from build123d import *

# Parameters (mm, degrees)
SKETCH1_W           = 32.3
SKETCH1_H           = 36.7
BOSS_EXTRUDE1_DEPTH = 1.5
SKETCH2_W           = 32.3
SKETCH2_H           = 1.5
BOSS_EXTRUDE2_DEPTH = 16.8
SKETCH3_W           = 22.7
SKETCH3_H           = 11.8
BOSS_EXTRUDE3_DEPTH = 3
SKETCH4_R           = 5.9
BOSS_EXTRUDE4_DEPTH = 4.3
SKETCH7_W           = 22.7
SKETCH7_H           = 11.8
BOSS_EXTRUDE6_DEPTH = 3
SKETCH9_R           = 5.9
BOSS_EXTRUDE7_DEPTH = 4.3
BOSS_EXTRUDE8_START = -1.5
SKETCH7_2_W         = 22.7
SKETCH7_2_H         = 11.8
BOSS_EXTRUDE8_DEPTH = 19
BOSS_EXTRUDE9_START = -20.5
SKETCH3_2_W         = 22.7
SKETCH3_2_H         = 11.8
BOSS_EXTRUDE9_DEPTH = 19


with BuildPart() as part:
    # Sketch1 → Boss-Extrude1 (new body)
    with BuildSketch(Plane.XY):
        Rectangle(SKETCH1_W, SKETCH1_H)
    extrude(amount=BOSS_EXTRUDE1_DEPTH)

    # Sketch2 → Boss-Extrude2 (add)
    with BuildSketch(Plane(origin=(0, 0, 0), x_dir=(-1, 0, 0), z_dir=(0, 0, -1))):
        with Locations((0, -17.6)):
            Rectangle(SKETCH2_W, SKETCH2_H)
    extrude(amount=BOSS_EXTRUDE2_DEPTH)

    # Sketch3 → Boss-Extrude3 (add)
    with BuildSketch(Plane.XZ.offset(18.35)):
        with Locations((-0.2, -8.9)):
            Rectangle(SKETCH3_W, SKETCH3_H)
    extrude(amount=BOSS_EXTRUDE3_DEPTH)

    # Sketch4 → Boss-Extrude4 (add)
    with BuildSketch(Plane.XZ.offset(21.35)):
        with BuildLine():
            ThreePointArc((-0.35, -6.307703721), (0.098043145, -7.56958653), (0.25, -8.9))
            ThreePointArc((0.25, -8.9), (0.098043145, -10.23041347), (-0.35, -11.492296279))
            ThreePointArc((-0.35, -11.492296279), (3.85, -8.9), (-0.35, -6.307703721))
        make_face()
        with Locations((-5.65, -8.9)):
            Circle(SKETCH4_R)
    extrude(amount=BOSS_EXTRUDE4_DEPTH)

    # Sketch7 → Boss-Extrude6 (add)
    with BuildSketch(Plane(origin=(-13.214346586, -22.528065204, 1.5), x_dir=(-1, 0, 0), z_dir=(0, 0, 1))):
        with Locations((-13.414346586, -31.978065204)):
            Rectangle(SKETCH7_W, SKETCH7_H)
    extrude(amount=BOSS_EXTRUDE6_DEPTH)

    # Sketch9 → Boss-Extrude7 (add)
    with BuildSketch(Plane(origin=(-13.214346586, -22.528065204, 4.5), x_dir=(-1, 0, 0), z_dir=(0, 0, 1))):
        with Locations((-7.964346586, -31.978065204)):
            Circle(SKETCH9_R)
        with BuildLine():
            ThreePointArc((-13.264346586, -34.570361484), (-13.864346586, -31.978065204), (-13.264346586, -29.385768925))
            ThreePointArc((-13.264346586, -29.385768925), (-17.464346586, -31.978065204), (-13.264346586, -34.570361484))
        make_face()
    extrude(amount=BOSS_EXTRUDE7_DEPTH)

    # Sketch7<2> → Boss-Extrude8 (add)
    with BuildSketch(Plane(origin=(-13.214346586, -22.528065204, 1.5), x_dir=(-1, 0, 0), z_dir=(0, 0, 1)).offset(BOSS_EXTRUDE8_START)):
        with Locations((-13.414346586, -31.978065204)):
            Rectangle(SKETCH7_2_W, SKETCH7_2_H)
    extrude(amount=-BOSS_EXTRUDE8_DEPTH)

    # Sketch3<2> → Boss-Extrude9 (add)
    with BuildSketch(Plane.XZ.offset(18.35).offset(BOSS_EXTRUDE9_START)):
        with Locations((-0.2, -8.9)):
            Rectangle(SKETCH3_2_W, SKETCH3_2_H)
    extrude(amount=BOSS_EXTRUDE9_DEPTH)


solid = part.part
Verification items for the finished model (mm, model axes). A direction names the side the tool comes from. Coordinates: 2 decimals unless noted, no trailing zeros. Loops run counter-clockwise (first coordinate to the right, second up) from the corner with the lowest first, then second, coordinate; pieces in that order, holes last. Notation, with made-up numbers: (14.25, -33) -> (71.25, -33) arc R20 cw to (71.25, -4) -> close; hole circle Ø6 at (89.5, 70). An arc over 180 degrees is marked (long way). Answer as a JSON object with one key per item and string values. Group by question number.
Item 1: Sectioned sample at B-B on x = 7. Record the boundary of the cut face in (y, z), plus the area to 3 significant figures.
Item 2: Tool access check on faces 4 (the flat face through (0, -18, -16.8)), 5 (the flat face through (11.55, 10, -9)), 6 (the cylindrical face through (-11.146, 9.672, 6.62)), 7 (the flat face through (11.15, -20, -9)), 8 (the flat face through (0, -7, -3)). Record the directions out of +Z, -Z, +X, -X, +Y, -Y that give a thin tool (end or side, any length) a straight path to the whole face; none if there is none.
Item 3: Scan lines: probe 1 along Z at (x, y) = (7.5, -5); probe 2 along Y at (x, z) = (4, -7.5); probe 3 along Y at (x, z) = (10.5, -1.5). Record each from-to range of solid material in increasing order.
Item 4: Sectioned sample at D-D on y = 13. Record the boundary of the cut face in (x, z).
Item 5: Sectioned sample at C-C on z = -13.5. Record the boundary of the cut face in (x, y), plus the area to 3 significant figures.
Item 6: Depth check by flat-ended pin: pin 1 (0.9 mm diameter, centred on y = 7, z = 3.5, fed in from -X); pin 2 (2 mm diameter, centred on y = 9, z = -7, fed in from +X); pin 3 (4 mm diameter, centred on x = 8, z = -8.5, fed in from -Y). Enter the tip coordinate at first touch or a pass-through.
Item 7: Sectioned sample at A-A on y = -3.5. Record the boundary of the cut face in (x, z), plus the area to 3 significant figures.
Item 8: Mould release check, pull along Y, two halves, no side actions. Record for faces 1 (the flat face through (0, -7, -14.8)), 2 (the flat face through (4, -21.35, -9)), 3 (the flat face through (0, 9, -19)): +Y half, -Y half, draft (parallel to the pull), parting line (faces both ways), or undercut.
Evaluation:
{
 "1": {"outline": "(-21.35, -14.8) -> (-18.35, -14.8) -> (-18.35, -16.8) -> (-16.85, -16.8) -> (-16.85, -14.8) -> (2.15, -14.8) -> (2.15, -3) -> (-16.85, -3) -> (-16.85, 0) -> (3.55, 0) -> (3.55, -19) -> (15.35, -19) -> (15.35, 0) -> (18.35, 0) -> (18.35, 1.5) -> (15.35, 1.5) -> (15.35, 4.5) -> (3.55, 4.5) -> (3.55, 1.5) -> (-18.35, 1.5) -> (-18.35, -3) -> (-21.35, -3) -> close", "area": "599 mm²"},
 "2": {"face 4": "-Z, +X, -X, -Y", "face 5": "-Z, +X, +Y", "face 6": "+Z", "face 7": "+Z, -Z, +X, -Y", "face 8": "+X, -X"},
 "3": {"probe 1": "z = -14.8 to -3, 0 to 1.5", "probe 2": "y = -21.35 to 2.15, 3.55 to 15.35", "probe 3": "y = -18.35 to -16.85, 3.55 to 15.35"},
 "4": {"outline": "(-16.15, 0) -> (-11.15, 0) -> (-11.15, -19) -> (11.55, -19) -> (11.55, 0) -> (16.15, 0) -> (16.15, 1.5) -> (11.55, 1.5) -> (11.55, 4.5) -> (-0.54, 4.5) -> (-0.54, 8.8) -> (-9.96, 8.8) -> (-9.96, 4.5) -> (-11.15, 4.5) -> (-11.15, 1.5) -> (-16.15, 1.5) -> close"},
 "5": {"outline": "(-16.15, -18.35) -> (-11.55, -18.35) -> (-11.55, -21.35) -> (-9.34, -21.35) -> (-9.34, -25.65) -> (-1.96, -25.65) -> (-1.96, -21.35) -> (11.15, -21.35) -> (11.15, -18.35) -> (16.15, -18.35) -> (16.15, -16.85) -> (11.15, -16.85) -> (11.15, 2.15) -> (-11.55, 2.15) -> (-11.55, -16.85) -> (-16.15, -16.85) -> close; (-11.15, 3.55) -> (11.55, 3.55) -> (11.55, 15.35) -> (-11.15, 15.35) -> close", "area": "847 mm²"},
 "6": {"pin 1": "stops at x = -11.15", "pin 2": "stops at x = 11.55", "pin 3": "stops at y = -21.35"},
 "7": {"outline": "(-16.15, 0) -> (16.15, 0) -> (16.15, 1.5) -> (-16.15, 1.5) -> close; (-11.55, -14.8) -> (11.15, -14.8) -> (11.15, -3) -> (-11.55, -3) -> close", "area": "316 mm²"},
 "8": {"face 1": "undercut", "face 2": "-Y half", "face 3": "draft"}
}
